from build123d import *

# Parameters (mm, degrees)
CHAMFER_1_SIZE      = 0.9
CHAMFER_1_SIZE2     = 0.630186784
CUT_EXTRUDE_1_DEPTH = 1.5
FILLET_1_R          = 0.4


with BuildPart() as part:
    # 草图2 → 旋转1 (revolve)
    with BuildSketch(Plane(origin=(0, 0, 0), x_dir=(0, 0, -1), z_dir=(1, 0, 0))):
        Polygon((0, 0), (0, 3.5), (1.8, 3.5), (1.8, 1.5), (9.8, 1.5), (9.8, 0), align=None)
    revolve(axis=Axis((0, 0, -9.8), (0, 0, 1)))

    # 倒角1
    chamfer_1_edges = [part.edges().sort_by_distance(p)[0] for p in [
        (0, -3.5, 0),
    ]]
    chamfer_1_side = [part.faces().sort_by_distance(p)[0] for p in [
        (0, 0, 0),
    ]]
    chamfer(chamfer_1_edges, length=CHAMFER_1_SIZE, length2=CHAMFER_1_SIZE2, reference=chamfer_1_side[0])

    # 草图3 → 切除-拉伸1 (cut)
    with BuildSketch(Plane.XY):
        Polygon((0.577350269, 1), (-0.577350269, 1), (-1.154700538, 0), (-0.577350269, -1), (0.577350269, -1), (1.154700538, 0), align=None)
    extrude(amount=-CUT_EXTRUDE_1_DEPTH, mode=Mode.SUBTRACT)

    # 圆角1
    fillet_1_edges = [part.edges().sort_by_distance(p)[0] for p in [
        (0, -3.5, -1.8),
    ]]
    fillet(fillet_1_edges, radius=FILLET_1_R)


solid = part.part
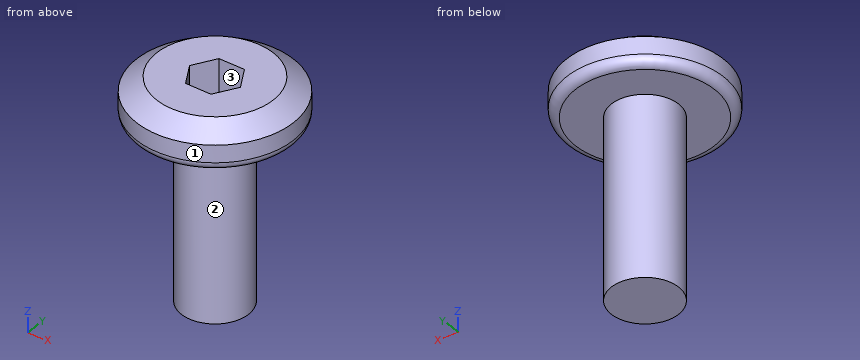
Geometry check sheet. Reference: the model listing, model coordinates, mm. Face numbers are marked on the shaded views. A direction names the side the tool comes from. Round coordinates to 2 decimals unless told otherwise and drop trailing zeros. Write each loop counter-clockwise with the first axis right and the second up, starting at its lowest first coordinate (ties: lowest second). Pieces come first, ordered by that corner, then holes. Notation, with made-up numbers: (39, 58) - (44, 58) arc R19 ccw to (44, 83) - close; hole circle Ø11 at (26, -10.75). An arc over 180 degrees is marked (long way). One line per item, written item: value.
1. Depth check by flat-ended pin: pin 1 Ø1.5 at (x, z) = (-2.5, -5) entering from +Y; pin 2 Ø0.6 at (x, y) = (0, 0) entering from +Z. Enter the tip coordinate at first touch or a pass-through.
The answers:
pin 1: passes through
pin 2: stops at z = -1.5
2. Set-up check for the marked faces 1, 2 and 3: record each of +Z, -Z, +X, -X, +Y, -Y from which the full face is reachable in a straight line by a thin tool's end or side.
The answers:
face 1: +Z, -Z
face 2: -Z
face 3: +Z
3. Scan lines: L1, parallel to Z at x = 1.5, y = 1.5; L2, parallel to Y at x = 0, z = -4.75; L3, parallel to X at y = 1, z = -2. Record each from-to range of solid material in increasing order.
The answers:
L1: z = -1.8 to 0
L2: y = -1.5 to 1.5
L3: x = -1.12 to 1.12
4. Cross-section at B-B on z = -6.25. Record the boundary of the cut face in (x, y).
The answers:
outline: circle Ø3 at (0, 0)
5. Cross-section at A-A on x = 0. Record the boundary of the cut face in (y, z).
The answers:
outline: (-3.5, -1.4) arc R0.4 ccw to (-3.1, -1.8) - (-1.5, -1.8) - (-1.5, -9.8) - (1.5, -9.8) - (1.5, -1.8) - (3.1, -1.8) arc R0.4 ccw to (3.5, -1.4) - (3.5, -0.63) - (2.6, 0) - (1, 0) - (1, -1.5) - (-1, -1.5) - (-1, 0) - (-2.6, 0) - (-3.5, -0.63) - close
